Could you check a few things on this model? Use its own coordinates, in mm. Coordinates: 2 decimals unless noted, no trailing zeros. Loops run counter-clockwise (first coordinate to the right, second up) from the corner with the lowest first, then second, coordinate; pieces in that order, holes last.
from build123d import *

# Parameters (mm, degrees)
TAP_DRILL_FOR_M6X1_0_TAP1_D     = 5
TAP_DRILL_FOR_M6X1_0_TAP1_DEPTH = 7
TAP_DRILL_FOR_M6X1_0_TAP1_TIP   = 1.502151548


with BuildPart() as part:
    # Sketch2 → Revolve1 (revolve)
    with BuildSketch(Plane(origin=(0, 0, 0), x_dir=(0, 0, -1), z_dir=(1, 0, 0))):
        Polygon((0, 0), (45.7, 0), (45.7, 5.5), (5, 5.5), (5, 4), (0, 4), align=None)
    revolve(axis=Axis((0, 0, 0), (0, 0, -1)))

    # Tap Drill for M6x1.0 Tap1
    with Locations(Plane(origin=(0, 0, -45.7), x_dir=(-1, 0, 0), z_dir=(0, 0, -1))):
        with Locations((0, 0)):
            Hole(TAP_DRILL_FOR_M6X1_0_TAP1_D / 2, depth=TAP_DRILL_FOR_M6X1_0_TAP1_DEPTH)
            with Locations((0, 0, -(TAP_DRILL_FOR_M6X1_0_TAP1_DEPTH + TAP_DRILL_FOR_M6X1_0_TAP1_TIP / 2))):  # 118° drill point
                Cone(0, TAP_DRILL_FOR_M6X1_0_TAP1_D / 2, TAP_DRILL_FOR_M6X1_0_TAP1_TIP, mode=Mode.SUBTRACT)


solid = part.part
(1) We'd pull the mould along Y, two halves only. Please class faces 1 (the face through (-3.905, -0.867, -2.465)), 2 (the face through (-0.54, -2.44, -42.15)), 3 (the face through (-2, -4, -5)): +Y half, -Y half, draft (parallel to the pull), parting line (faces both ways), or undercut.
Answers:
face 1: parting line
face 2: undercut
face 3: draft
(2) I need wall thicknesses on probe 1 along X at (y, z) = (0, -43.5); probe 2 along Z at (x, y) = (2.25, 3.5); probe 3 along Y at (x, z) = (2, -41.5). Which ranges of each line are inside material? Lowest first, please.
Answers:
probe 1: x = -5.5 to -2.5, 2.5 to 5.5
probe 2: z = -45.7 to -5
probe 3: y = -5.12 to -1.5, 1.5 to 5.12
(3) For pin 1 (2 mm diameter, centred on x = 3, z = -37.5, fed in from +Y); pin 2 (3 mm diameter, centred on y = -4.5, z = -32.5, fed in from +X), each with a flat end and sliding along its axis, tell me the tip position at first contact or that it passes through.
Answers:
pin 1: stops at y = 5.12
pin 2: stops at x = 4.61
(4) Imagine slicing it at B-B, the plane z = -41.5. Write out the boundary of the cut face in (x, y), and give its area (3 significant figures).
Answers:
outline: circle Ø11 at (0, 0); hole circle Ø5 at (0, 0)
area: 75.4 mm2
(5) Imagine slicing it at A-A, the plane z = -30. Write out the boundary of the cut face in (x, y), and give its area (3 significant figures).
Answers:
outline: circle Ø11 at (0, 0)
area: 95.0 mm2
